Can you work these out from the model? Positions are in its coordinate system, mm. A direction names the side the tool comes from. Coordinates: 2 decimals unless noted, no trailing zeros. Loops run counter-clockwise (first coordinate to the right, second up) from the corner with the lowest first, then second, coordinate; pieces in that order, holes last. Notation, with made-up numbers: (67.25, 17.5) -> (125.25, 17.5) arc R21 ccw to (125.25, 24.5) -> close; hole circle Ø2 at (58.5, 9.5). An arc over 180 degrees is marked (long way). Put each result on its own line as item: value. Start each with the question number.
Item 1: Please list where these lines run through material, in increasing order: L1, parallel to X at y = -33, z = -32.5; L2, parallel to Z at x = 44, y = -11; L3, parallel to Z at x = 58.65, y = 0. Write a range as from..to.
Item 2: We'd pull the mould along Y, two halves only. Please class faces 1 (the flat face through (59, 9, 1)), 2 (the flat face through (29, -37, 1)), 3 (the cylindrical face through (57.99, -4.88, 1.08)): pulls with the +Y half, pulls with the -Y half, needs draft (parallel to the pull), parting line crosses it, or undercut.
Item 3: Will this pin go through, and if not, where does the flat tip stop? P1, Ø9, axis at y = 0, z = 0, coming from the +X side.
Item 4: If we section it at C-C on x = 14.5: Please give me the cut outline in (y, z).
Item 5: If we section it at A-A on z = 0: Please give me the cut outline in (x, y).
Item 6: If we section it at B-B on y = -26: Please give me the cut outline in (x, z).
Item 7: For faces 4 (the flat face through (29, -1, -40.5)), 5 (the flat face through (29, 35, -1)), which set-ups out of +Z, -Z, +X, -X, +Y, -Y let a thin tool reach every point of the face, with its end or its side?
Item 8: If we section it at D-D on y = 0: Please give me the cut outline in (x, z).
```python
from build123d import *

# Parameters (mm, degrees)
SKETCH1_W           = 81
SKETCH1_H           = 74
BOSS_EXTRUDE1_DEPTH = 59
SKETCH3_R           = 5
CUT_EXTRUDE1_DEPTH  = 160
SKETCH4_W           = 55
SKETCH4_H           = 77
CUT_EXTRUDE2_DEPTH  = 70


with BuildPart() as part:
    # Sketch1 → Boss-Extrude1 (new body)
    with BuildSketch(Plane(origin=(0, 0, 0), x_dir=(0, 0, -1), z_dir=(1, 0, 0))):
        Rectangle(SKETCH1_W, SKETCH1_H)
    extrude(amount=BOSS_EXTRUDE1_DEPTH)

    # Sketch3 → Cut-Extrude1 (cut)
    with BuildSketch(Plane(origin=(0, 0, 0), x_dir=(0, 0, -1), z_dir=(1, 0, 0))):
        Circle(SKETCH3_R)
    extrude(amount=CUT_EXTRUDE1_DEPTH, mode=Mode.SUBTRACT)

    # Sketch4 → Cut-Extrude2 (cut)
    with BuildSketch(Plane(origin=(0, 35, 0), x_dir=(1, 0, 0), z_dir=(0, 1, 0))):
        with Locations((29.5, 0)):
            Rectangle(SKETCH4_W, SKETCH4_H)
    extrude(amount=-CUT_EXTRUDE2_DEPTH, mode=Mode.SUBTRACT)


solid = part.part
```
Solutions:
1. L1: 0..2, 57..59
1. L2: -40.5..-38.5, 38.5..40.5
1. L3: -40.5..-5, 5..40.5
2. face 1: needs draft
2. face 2: pulls with the -Y half
2. face 3: undercut
3. P1: through
4. outline: (-37, -40.5) -> (37, -40.5) -> (37, 40.5) -> (-37, 40.5) -> close; hole (-35, -38.5) -> (35, -38.5) -> (35, 38.5) -> (-35, 38.5) -> close
5. outline: (0, -37) -> (59, -37) -> (59, -5) -> (57, -5) -> (57, -35) -> (2, -35) -> (2, -5) -> (0, -5) -> close; (0, 5) -> (2, 5) -> (2, 35) -> (57, 35) -> (57, 5) -> (59, 5) -> (59, 37) -> (0, 37) -> close
6. outline: (0, -40.5) -> (59, -40.5) -> (59, 40.5) -> (0, 40.5) -> close; hole (2, -38.5) -> (57, -38.5) -> (57, 38.5) -> (2, 38.5) -> close
7. face 4: -Z, +X, -X, +Y, -Y
7. face 5: none
8. outline: (0, -40.5) -> (59, -40.5) -> (59, -5) -> (57, -5) -> (57, -38.5) -> (2, -38.5) -> (2, -5) -> (0, -5) -> close; (0, 5) -> (2, 5) -> (2, 38.5) -> (57, 38.5) -> (57, 5) -> (59, 5) -> (59, 40.5) -> (0, 40.5) -> close
